Geometry check sheet. Reference: the model listing, model coordinates, mm. A direction names the side the tool comes from. Give positions to 0.01 mm unless a question says otherwise; leave off trailing zeros. Write each loop counter-clockwise with the first axis right and the second up, starting at its lowest first coordinate (ties: lowest second). Pieces come first, ordered by that corner, then holes. Notation, with made-up numbers: M -39,-8.5 L -32,-8.5 A14 cw -32,8.5 Z; hole C -8,24 d3. An arc over 180 degrees is marked long. One line per item, written item: value. Start each with the question number.
1. Tool access check on faces 5 (the face through (4.5, 9, 11)), 6 (the face through (5, 9, 12)), 7 (the face through (-0.1, 27, 3.3)), 8 (the face through (6, 9, 11)). Record the directions out of +Z, -Z, +X, -X, +Y, -Y that give a thin tool (end or side, any length) a straight path to the whole face; none if there is none.
2. Cross-section at B-B on z = 0. Record the cut outline in (x, y), then the cut area to 3 significant figures.
3. Cross-section at D-D on x = -3.5. Record the cut outline in (y, z).
4. Cross-section at A-A on y = 5. Record the cut outline in (x, z), then the cut area to 3 significant figures.
5. Release check for a two-part mould opening along X. For faces 1 (the face through (0, 9, -11)), 2 (the face through (-4.5, 9, 11)), 3 (the face through (-6, 9, 11)), 4 (the face through (0, 39, 0)) record: pulls with the +X half, pulls with the -X half, needs draft (parallel to the pull), parting line crosses it, or undercut.
6. Scan lines: line 1 (X direction, y = 7, z = 11.25); line 2 (Y direction, x = -1.5, z = -5); line 3 (Y direction, x = -1.5, z = -4.5). Record each from-to range of solid material in increasing order.
7. Gauge pin test, flat ends, axial feed: pin 1 (3 mm diameter, centred on x = -2, y = 29.5, fed in from -Z); pin 2 (3 mm diameter, centred on y = 26.5, z = 5.5, fed in from +X); pin 3 (2 mm diameter, centred on y = 14, z = 10.5, fed in from -X); pin 4 (3 mm diameter, centred on y = 7.5, z = 1, fed in from -X). Record the tip position at first contact, or that the pin passes through.
8. Cross-section at C-C on x = 0. Record the cut outline in (y, z), then the cut area to 3 significant figures.
from build123d import *

# Parameters (mm, degrees)
BOSS_EXTRUDE1_DEPTH = 19
SKETCH2_R           = 5
BOSS_EXTRUDE2_DEPTH = 8
SKETCH3_R           = 3
BOSS_EXTRUDE3_DEPTH = 12


with BuildPart() as part:
    # Sketch1 → Boss-Extrude1 (new body)
    with BuildSketch(Plane(origin=(0, 0, 0), x_dir=(1, 0, 0), z_dir=(0, 1, 0))):
        with BuildLine():
            Line((-6, -12), (-4.5, -12))
            Line((-4.5, -12), (-4.5, -10.03742995))
            ThreePointArc((-4.5, -10.03742995), (0, -11), (4.5, -10.03742995))
            Line((4.5, -10.03742995), (4.5, -12))
            Line((4.5, -12), (6, -12))
            Line((6, -12), (6, -9.219544457))
            ThreePointArc((6, -9.219544457), (0, 11), (-6, -9.219544457))
            Line((-6, -9.219544457), (-6, -12))
        make_face()
    extrude(amount=BOSS_EXTRUDE1_DEPTH)

    # Sketch2 → Boss-Extrude2 (add)
    with BuildSketch(Plane(origin=(0, 19, 0), x_dir=(1, 0, 0), z_dir=(0, 1, 0))):
        Circle(SKETCH2_R)
    extrude(amount=BOSS_EXTRUDE2_DEPTH)

    # Sketch3 → Boss-Extrude3 (add)
    with BuildSketch(Plane(origin=(0, 27, 0), x_dir=(1, 0, 0), z_dir=(0, 1, 0))):
        Circle(SKETCH3_R)
    extrude(amount=BOSS_EXTRUDE3_DEPTH)


solid = part.part
Report:
1. face 5: +Z, +Y, -Y
1. face 6: +Z, +X, -X, +Y, -Y
1. face 7: +Y
1. face 8: +Z, +X, +Y, -Y
2. outline: M -11,0 L 11,0 L 11,19 L 5,19 L 5,27 L 3,27 L 3,39 L -3,39 L -3,27 L -5,27 L -5,19 L -11,19 Z
2. area: 570 mm^2
3. outline: M 0,-10.43 L 19,-10.43 L 19,-3.57 L 27,-3.57 L 27,3.57 L 19,3.57 L 19,10.43 L 0,10.43 Z
4. outline: M -6,9.22 A11 ccw long 6,9.22 L 6,12 L 4.5,12 L 4.5,10.04 A11 ccw -4.5,10.04 L -4.5,12 L -6,12 Z
4. area: 387 mm^2
5. face 1: parting line crosses it
5. face 2: undercut
5. face 3: pulls with the -X half
5. face 4: needs draft
6. line 1: x = -6 to -4.5, 4.5 to 6
6. line 2: y = 0 to 19
6. line 3: y = 0 to 27
7. pin 1: stops at z = -2.96
7. pin 2: stops at x = 3
7. pin 3: stops at x = -6
7. pin 4: stops at x = -11
8. outline: M 0,-11 L 19,-11 L 19,-5 L 27,-5 L 27,-3 L 39,-3 L 39,3 L 27,3 L 27,5 L 19,5 L 19,11 L 0,11 Z
8. area: 570 mm^2
